Model file for the job. Use its own axes, mm. A direction names the side the tool comes from. Round coordinates to 2 decimals unless told otherwise and drop trailing zeros. Loops run counter-clockwise (first coordinate to the right, second up) from the corner with the lowest first, then second, coordinate; pieces in that order, holes last. Notation, with made-up numbers: (-17.75, -35) -> (37.25, -35) arc R23 ccw to (37.25, 3) -> close; hole circle Ø2 at (70.5, -7). An arc over 180 degrees is marked (long way). Use a Markdown table: item, result. Add a question column.
```python
from build123d import *

# Parameters (mm, degrees)
F1_DEPTH    = 3.81
F3_T1_DEPTH = 111.8036914576
F4_DEPTH    = 1.27
F5_R        = 11.1870112164
F5_R_2      = 9.3121919152
F6_DEPTH    = 133.604
F7_R        = 25.2769928265
F7_R_2      = 11.1870112164
F7_R_3      = 9.3121919152
F8_DEPTH    = 25.4
F9_SIZE     = 12.7
F10_SIZE    = 5.08


# Not quite as in the source:
# - a fillet or chamfer that OpenCascade refuses, or shapes differently, is made with other operations: its cross-section is extruded or revolved along the edge and cut away or added


with BuildPart() as f1:
    # F0 (on Top) → F1 (new body)
    with BuildSketch(Plane.XY):
        with BuildLine():
            Line((45.1586060226, -52.2380582988), (26.3960231096, 43.0443435907))
            ThreePointArc((26.3960231096, 43.0443435907), (-2.1687844347, 58.4802777375), (-27.4601764977, 38.1194874644))
            Line((-27.4601764977, 38.1194874644), (-40.5167862773, -52.2380582988))
            Line((-40.5167862773, -52.2380582988), (45.1586060226, -52.2380582988))
        make_face()
    extrude(amount=F1_DEPTH)

    # F3: chamfer of 5.08 on 1 edges, made by hand

    # F3_s2 → F3_t1 (cut)
    with BuildSketch(Plane.YZ.offset(-53.5809358562)):
        Polygon((-52.2380582988, -1.27), (-47.1580582988, 3.81), (-52.2380582988, 3.81), align=None)
    extrude(amount=F3_T1_DEPTH, mode=Mode.SUBTRACT)

    # F2 (on face) → F4 (join)
    with BuildSketch(Plane.XY.offset(3.81)):
        with BuildLine():
            ThreePointArc((26.3960231096, 43.0443435907), (-2.1687844347, 58.4802777375), (-27.4601764977, 38.1194874644))
            ThreePointArc((-27.4601764977, 38.1194874644), (0.9757940306, 24.0924618975), (26.3960231096, 43.0443435907))
        make_face()
    extrude(amount=F4_DEPTH)

    # F5 (on face) → F6 (join)
    with BuildSketch(Plane.XY.offset(5.08)):
        with Locations((0, 40.8166870475)):
            Circle(F5_R)
        with Locations((0, 40.8166870475)):
            Circle(F5_R_2, mode=Mode.SUBTRACT)
    extrude(amount=F6_DEPTH)

    # F7 (on face) → F8 (join)
    with BuildSketch(Plane.XY.offset(138.684)):
        with Locations((0, 40.8166870475)):
            Circle(F7_R)
        with Locations((0, 40.8166870475)):
            Circle(F7_R_2, mode=Mode.SUBTRACT)
        with Locations((0, 40.8166870475)):
            Circle(F7_R_2)
        with Locations((0, 40.8166870475)):
            Circle(F7_R_3, mode=Mode.SUBTRACT)
    extrude(amount=F8_DEPTH)

    # F9
    f9_edges = [f1.edges().sort_by_distance(p)[0] for p in [
        (-25.276993, 40.816687, 138.684),
    ]]
    chamfer(f9_edges, length=F9_SIZE)

    # F10
    f10_edges = [f1.edges().sort_by_distance(p)[0] for p in [
        (-25.276993, 40.816687, 151.384),
    ]]
    chamfer(f10_edges, length=F10_SIZE)


solid = f1.part
```
1) Pin check, flat tips, straight feed: pin 1 Ø15 at (x, y) = (0, 40.82) entering from +Z; pin 2 Ø5 at (x, z) = (15.5, 84) entering from -Y; pin 3 Ø1 at (x, z) = (3, 130) entering from -Y; pin 4 Ø1 at (x, y) = (-18.5, -3) entering from +Z. Stop position of each tip, or through.
2) Tool access for faces 5 (the face through (-1.69, 58.52, 2.5)), 6 (the face through (0.51, 24.054, 4.436)), 7 (the face through (-8, 32, 138.684)), 8 (the face through (5.006, 48.669, 83.469)): list every direction of +Z, -Z, +X, -X, +Y, -Y with a clear straight run to the whole face (end or side of a thin tool).
3) Wall check: probe 1 along Y at (x, z) = (0, 96); probe 2 along Z at (x, y) = (5, 3.5); probe 3 along Z at (x, y) = (14, 33). Give the ranges that are in metal, low to high. Write a range as from..to.
4) Cut at B-B on y = -16. Write the cut outline in (x, z), and give its area (3 significant figures).
5) Cut at A-A on z = 20.5. Write the cut outline in (x, y), and give its area (3 significant figures).
6) Pull direction Y, two halves, no side cores. Call faces 1 (the face through (1.69, -49.09, 1.88)), 2 (the face through (-3.29, 65.88, 160.22)), 3 (the face through (0, 41, 5.08)), 4 (the face through (2, -11, 3.81)): +Y half, -Y half, draft (parallel to the pull), parting line (faces both ways), or undercut.
Established:
| question | item | result |
|---|---|---|
| 1 | pin 1 | stops at z = 5.08 |
| 1 | pin 2 | passes through |
| 1 | pin 3 | stops at y = 29.91 |
| 1 | pin 4 | stops at z = 3.81 |
| 2 | face 5 | -Z, +Y |
| 2 | face 6 | -Y |
| 2 | face 7 | none |
| 2 | face 8 | +Z |
| 3 | probe 1 | y = 29.63..31.5, 50.13..52 |
| 3 | probe 2 | z = 0..3.81 |
| 3 | probe 3 | z = 0..5.08, 142.14..164.08 |
| 4 | outline | (-35.28, 0) -> (38.02, 0) -> (38.02, 3.81) -> (-35.28, 3.81) -> close |
| 4 | area | 279 mm^2 |
| 5 | outline | circle Ø22.37 at (0, 40.82); hole circle Ø18.62 at (0, 40.82) |
| 5 | area | 121 mm^2 |
| 6 | face 1 | -Y half |
| 6 | face 2 | parting line |
| 6 | face 3 | undercut |
| 6 | face 4 | draft |
